Read the model definition and answer for the solid it produces. Units are mm, in the model's axes. A direction names the side the tool comes from. Coordinates: 2 decimals unless noted, no trailing zeros. Order: outer loops, then holes, each group sorted by start corner. A loop starts at its lowest first (then second) coordinate and runs counter-clockwise, first axis right, second up. Notation, with made-up numbers: (40.5, -39) - (76.5, -39) arc R31 cw to (76.5, -15) - close; hole circle Ø4 at (40.25, 60). An arc over 180 degrees is marked (long way). Use one line per item in the form item = value.
```python
from build123d import *

# Parameters (mm, degrees)
F0_W     = 30
F0_H     = 45
F0_H_2   = 10
F1_DEPTH = 30
F3_DEPTH = 30.001
F4_W     = 2.6
F4_H     = 31.6227766017
F5_DEPTH = 3
F7_DEPTH = 2.6


with BuildPart() as f1:
    # F0 (on Top) → F1 (new body)
    with BuildSketch(Plane.XY):
        Rectangle(F0_W, F0_H)
        with Locations((0, -27.5)):
            Rectangle(F0_W, F0_H_2)
    extrude(amount=F1_DEPTH)

    # F2 (on face) → F3 (cut, through all)
    with BuildSketch(Plane.YZ.offset(15)):
        Polygon((-32.5, 0), (-22.5, 0), (-32.5, 30), align=None)
        Polygon((22.5, 30), (-32.5, 30), (22.5, 0), align=None)
    extrude(amount=-F3_DEPTH, mode=Mode.SUBTRACT)

    # F4 (on face) → F5 (cut)
    with BuildSketch(Plane(origin=(0, -20.25, -6.75), x_dir=(1, 0, 0), z_dir=(0, -0.9486832981, -0.316227766))):
        with Locations((13.7, 22.9265130362)):
            Rectangle(F4_W, F4_H)
    extrude(amount=-F5_DEPTH, mode=Mode.SUBTRACT)

    # F6 (on face) → F7 (cut)
    with BuildSketch(Plane.YZ.offset(15)):
        Polygon((-19.6539501058, 0), (-19.6539501058, 0.9486832981), (-22.5, 0), align=None)
    extrude(amount=-F7_DEPTH, mode=Mode.SUBTRACT)


solid = f1.part
```
(1) Straight lines are drawn through the part: L1, parallel to Z at x = 1.5, y = -22; L2, parallel to Z at x = -3, y = 13.5; L3, parallel to Y at x = -5, z = 12.5. For each, find the intervals that lie inside material, in ascending order.
Answer list:
L1 = 0 to 24.27
L2 = 0 to 4.91
L3 = -26.67 to -0.42
(2) Section D-D, the plane x = 13.5 is taken. Write down the section's boundary in (y, z) (3 decimals), then the cut area to 3 significant figures.
Answer list:
outline = (-28.635, 27.892) - (-19.654, 0.949) - (-19.654, 0) - (22.5, 0) - close
area = 584 mm2
(3) Given pin 1 Ø2 at (x, y) = (7, -12.5) entering from +Z; pin 2 Ø4 at (y, z) = (-27, 16) entering from +X; pin 3 Ø5 at (x, y) = (-4.5, -18.5) entering from +Z, each flat-ended and moving along its own axis, determine where each tip first touches the part or whether it passes through.
Answer list:
pin_1 = 19.64
pin_2 = 12.4
pin_3 = 23.73
(4) Section B-B, the plane z = 3 is taken. Write down the section's boundary in (x, y), then the cut area to 3 significant figures.
Answer list:
outline = (-15, -23.5) - (12.4, -23.5) - (12.4, -20.34) - (15, -20.34) - (15, 17) - (-15, 17) - close
area = 1,210 mm2
(5) Section A-A, the plane x = 2 is taken. Write down the section's boundary in (y, z).
Answer list:
outline = (-32.5, 30) - (-22.5, 0) - (22.5, 0) - close
(6) Section C-C, the plane y = -21 is taken. Write down the section's boundary in (x, z).
Answer list:
outline = (-15, 0) - (12.4, 0) - (12.4, 4.99) - (15, 4.99) - (15, 23.73) - (-15, 23.73) - close
(7) Which of the six approach directions +Z, -Z, +X, -X, +Y, -Y give full straight-line access (tool end or side, diameter ignored) to faces 1 (the flat face through (13.682, -24.207, 14.609)), 2 (the flat face through (15, -9, 11))?
Answer list:
face_1 = -Z, +X, -Y
face_2 = +Z, -Z, +X, +Y, -Y
